Could you check a few things on this model? Use its own coordinates, in mm. A direction names the side the tool comes from. Coordinates: 2 decimals unless noted, no trailing zeros. Loops run counter-clockwise (first coordinate to the right, second up) from the corner with the lowest first, then second, coordinate; pieces in that order, holes last.
Autodesk Inventor part; units mm, degrees
ref_plane "YZ Plane" through (0, 0, 0) normal (1, 0, 0) x (0, 1, 0)
ref_plane "XZ Plane" through (0, 0, 0) normal (0, 1, 0) x (-1, 0, 0)
ref_plane "XY Plane" through (0, 0, 0) normal (0, 0, 1) x (1, 0, 0)
sketch "Sketch_1" plane through (0, 0, 0) normal (1, 0, 0) x (0, 1, 0)
  line L0 (0, 50.8) -> (0, 0)
  line L1 (0, 0) -> (25.4, 0)
  arc A0 (25.4, 0) -> (20.6248, 4.7752) centre (20.6248, 0) ccw
  line L2 (20.6248, 4.7752) -> (7.9502, 4.7752)
  arc A1 (4.7752, 7.9502) -> (7.9502, 4.7752) centre (7.9502, 7.9502) ccw
  line L3 (4.7752, 7.9502) -> (4.7752, 46.0248)
  arc A2 (4.7752, 46.0248) -> (0, 50.8) centre (0, 46.0248) ccw
extrude "Extrusion1" add sketch "Sketch_1" along normal mid plane 22.225
sketch "Sketch2" plane through (11.1125, 25.4, 0) normal (0, 0, -1) x (-1, 0, 0)
  point P0 (11.1125, -12.7)
hole "Hole1" at (0, 12.7, 0) direction (0, 0, 1) diameter 7.1374 depth 4.7752
sketch "Sketch3" plane through (-11.1125, 0, 0) normal (0, -1, 0) x (1, 0, 0)
  point P0 (11.1125, 12.7)
hole "Hole2" at (0, 0, 12.7) direction (0, 1, 0) diameter 7.1374 depth 4.7752
sketch "Sketch4" plane through (-11.1125, 0, 0) normal (0, -1, 0) x (1, 0, 0)
  point P0 (11.1125, 38.1)
hole "Hole3" at (0, 0, 38.1) direction (0, 1, 0) diameter 7.1374 depth 4.7752
properties part number "4176"
(1) We'd pull the mould along Z, two halves only. Please class faces 3 (the face through (-1.072, 2.421, 34.696)), 4 (the face through (-0.157, 2.421, 16.265)), 5 (the face through (-0.16, 3.34, 49.44)), 6 (the face through (-3, 10, 0)): +Z half, -Z half, draft (parallel to the pull), parting line (faces both ways), or undercut.
Answers:
face 3: undercut
face 4: undercut
face 5: +Z half
face 6: -Z half
(2) Which directions (+Z, -Z, +X, -X, +Y, -Y) give clear straight access to the entire face, cutting with the end or side of a thin tool? Please do faces 1 (the face through (0, 17, 4.775)), 2 (the face through (0, 0, 26)).
Answers:
face 1: +Z, +X, -X, +Y
face 2: +Z, -Z, +X, -X, -Y
(3) Imagine slicing it at B-B, the plane x = 0. Write out the boundary of the cut face in (y, z) (3 decimals).
Answers:
outline: (0, 0) - (9.131, 0) - (9.131, 4.775) - (7.95, 4.775) arc R3.175 cw to (4.775, 7.95) - (4.775, 9.131) - (0, 9.131) - close; (0, 16.269) - (4.775, 16.269) - (4.775, 34.531) - (0, 34.531) - close; (0, 41.669) - (4.775, 41.669) - (4.775, 46.025) arc R4.775 ccw to (0, 50.8) - close; (16.269, 0) - (25.4, 0) arc R4.775 ccw to (20.625, 4.775) - (16.269, 4.775) - close
(4) I need wall thicknesses on probe 1 along X at (y, z) = (3.35, 38.1); probe 2 along Z at (x, y) = (0, 2.25); probe 3 along Z at (x, y) = (0, 2.5). Which ranges of each line are inside material? Lowest first, please.
Answers:
probe 1: x = -11.11 to -3.57, 3.57 to 11.11
probe 2: z = 0 to 9.13, 16.27 to 34.53, 41.67 to 50.24
probe 3: z = 0 to 9.13, 16.27 to 34.53, 41.67 to 50.09
(5) Imagine slicing it at D-D, the plane x = -6.25. Write out the boundary of the cut face in (y, z) (3 decimals).
Answers:
outline: (0, 0) - (25.4, 0) arc R4.775 ccw to (20.625, 4.775) - (7.95, 4.775) arc R3.175 cw to (4.775, 7.95) - (4.775, 46.025) arc R4.775 ccw to (0, 50.8) - close
(6) Imagine slicing it at A-A, the plane z = 38.1. Write out the boundary of the cut face in (x, y), and give its area (3 significant figures).
Answers:
outline: (-11.11, 0) - (-3.57, 0) - (-3.57, 4.78) - (-11.11, 4.78) - close; (3.57, 0) - (11.11, 0) - (11.11, 4.78) - (3.57, 4.78) - close
area: 72.0 mm2
(7) For pin 1 (10 mm diameter, centred on y = 13.5, z = 10.5, fed in from +X); pin 2 (10 mm diameter, centred on x = -5.5, z = 11, fed in from +Y); pin 3 (11 mm diameter, centred on x = 2, z = 26, fed in from +Y), each with a flat end and sliding along its axis, tell me the tip position at first contact or that it passes through.
Answers:
pin 1: passes through
pin 2: stops at y = 5.44
pin 3: stops at y = 4.78
